Read the model definition and answer for the solid it produces. Units are mm, in the model's axes. A direction names the side the tool comes from. Coordinates: 2 decimals unless noted, no trailing zeros. Write each loop counter-clockwise with the first axis right and the second up, starting at its lowest first coordinate (ties: lowest second). Pieces come first, ordered by that corner, then holes.
1) Each of these flat-tipped pins is pushed along its axis until it touches: pin 1 Ø2 at (y, z) = (39.5, 4) entering from +X; pin 2 Ø3 at (x, z) = (29.5, 3.5) entering from +Y; pin 3 Ø1 at (x, z) = (48.5, 4.5) entering from +Y. Where does it stop, or does it pass through?
2) Determine the mould class of faces 1 (the face through (-56.01, -75.65, 3.13)), 2 (the face through (20, 1, 0)), 3 (the face through (-40.53, -26.39, 3.22)) for opening direction X: +X half, -X half, draft (parallel to the pull), parting line (faces both ways), or undercut.
3) Which of the six approach directions +Z, -Z, +X, -X, +Y, -Y give full straight-line access (tool end or side, diameter ignored) to faces 4 (the face through (20, 1, 6.35)), 5 (the face through (-27.13, -41.27, 3.22))?
4) Find the intervals of material crossed by line 1 (Y direction, x = 0, z = 5.25); line 2 (X direction, y = -38.5, z = 3.5); line 3 (X direction, y = -14, z = 2), in increasing order.
5) The part is cut by section A-A (z = 4.25). Determine the outline of the cut face in (x, y) (1 decimal), then the cut area to 3 significant figures.
6) The part is cut by section D-D (y = 27.5). Determine the outline of the cut face in (x, z).
7) The part is cut by section C-C (x = 58). Determine the outline of the cut face in (y, z), then the cut area to 3 significant figures.
8) The part is cut by section B-B (y = -41). Determine the outline of the cut face in (x, z).
from build123d import *

# Parameters (mm, degrees)
SKETCH1_R           = 97.5
SKETCH1_R_2         = 4.7625
SKETCH1_R_3         = 1.7859375
BOSS_EXTRUDE1_DEPTH = 6.35
CUT_EXTRUDE3_REACH  = 140.032
FILLET2_R           = 10
FILLET3_R           = 2.5


with BuildPart() as part:
    # Sketch1 → Boss-Extrude1 (new body)
    with BuildSketch(Plane.XY):
        Circle(SKETCH1_R)
        Circle(SKETCH1_R_2, mode=Mode.SUBTRACT)
        with Locations((0, 92.5)):
            Circle(SKETCH1_R_3, mode=Mode.SUBTRACT)
        with Locations((92.5, 0)):
            Circle(SKETCH1_R_3, mode=Mode.SUBTRACT)
        with Locations((0, -92.5)):
            Circle(SKETCH1_R_3, mode=Mode.SUBTRACT)
        with Locations((-92.5, 0)):
            Circle(SKETCH1_R_3, mode=Mode.SUBTRACT)
    extrude(amount=BOSS_EXTRUDE1_DEPTH)

    # Sketch5 → Cut-Extrude3 (cut, up to next)
    with BuildSketch(Plane.XY.offset(6.35), mode=Mode.PRIVATE) as cut_extrude3_sk1:
        with BuildLine():
            Line((1.414213562, -12.727922061), (-5.656854249, -5.656854249))
            Line((-5.656854249, -5.656854249), (-68.942911166, -68.942911166))
            ThreePointArc((-68.942911166, -68.942911166), (-65.311752388, -72.392161178), (-61.50826581, -75.650401434))
            Line((-61.50826581, -75.650401434), (1.414213562, -12.727922061))
        make_face()
    cut_extrude3_tool1 = extrude(cut_extrude3_sk1.sketch, amount=-CUT_EXTRUDE3_REACH, mode=Mode.PRIVATE) & part.part
    # Sketch5 → Cut-Extrude3 (cut, up to next)
    with BuildSketch(Plane.XY.offset(6.35), mode=Mode.PRIVATE) as cut_extrude3_sk2:
        with BuildLine():
            Line((-68.942911166, -68.942911166), (-5.656854249, -5.656854249))
            Line((-5.656854249, -5.656854249), (-12.727922061, 1.414213562))
            Line((-12.727922061, 1.414213562), (-75.650401434, -61.50826581))
            ThreePointArc((-75.650401434, -61.50826581), (-72.392161178, -65.311752388), (-68.942911166, -68.942911166))
        make_face()
    cut_extrude3_tool2 = extrude(cut_extrude3_sk2.sketch, amount=-CUT_EXTRUDE3_REACH, mode=Mode.PRIVATE) & part.part
    add(cut_extrude3_tool1.solids().sort_by_distance((-33.7073, -40.771587, 6.35))[0], mode=Mode.SUBTRACT)
    add(cut_extrude3_tool2.solids().sort_by_distance((-40.771587, -33.7073, 6.35))[0], mode=Mode.SUBTRACT)

    # Fillet2
    fillet2_edges = [part.edges().sort_by_distance(p)[0] for p in [
        (-61.50826581, -75.650401434, 3.175),
        (-75.650401434, -61.50826581, 3.175),
    ]]
    fillet(fillet2_edges, radius=FILLET2_R)

    # Fillet3
    fillet3_edges = [part.edges().sort_by_distance(p)[0] for p in [
        (-12.727922061, 1.414213562, 3.175),
        (1.414213562, -12.727922061, 3.175),
    ]]
    fillet(fillet3_edges, radius=FILLET3_R)


solid = part.part
Reported:
1. pin 1: stops at x = 89.58
1. pin 2: stops at y = 93.39
1. pin 3: stops at y = 84.87
2. face 1: -X half
2. face 2: draft
2. face 3: undercut
3. face 4: +Z, +X, -X, +Y, -Y
3. face 5: +Z, -Z
4. line 1: y = -97.5 to -94.29, -90.71 to -14.05, -11.41 to -4.76, 4.76 to 90.71, 94.29 to 97.5
4. line 2: x = -89.58 to -52.64, -24.36 to 89.58
4. line 3: x = -96.49 to -28.14, 0.03 to 96.49
5. outline: (-82.9, -51.4) arc R10 ccw to (-67.3, -53.2) - (-14.5, -0.4) arc R2.5 cw to (-11, -0.4) - (-0.4, -11) arc R2.5 cw to (-0.4, -14.5) - (-53.2, -67.3) arc R10 ccw to (-51.4, -82.9) arc R97.5 ccw (long way) to start; hole circle Ø3.6 at (-92.5, 0); hole circle Ø9.5 at (0, 0); hole circle Ø3.6 at (0, -92.5); hole circle Ø3.6 at (0, 92.5); hole circle Ø3.6 at (92.5, 0)
5. area: 27,900 mm2
6. outline: (-93.54, 0) - (93.54, 0) - (93.54, 6.35) - (-93.54, 6.35) - close
7. outline: (-78.37, 0) - (78.37, 0) - (78.37, 6.35) - (-78.37, 6.35) - close
7. area: 995 mm2
8. outline: (-88.46, 0) - (-55.14, 0) - (-55.14, 6.35) - (-88.46, 6.35) - close; (-26.86, 0) - (88.46, 0) - (88.46, 6.35) - (-26.86, 6.35) - close
